from build123d import *

# Parameters (mm, degrees)
SKETCH1_R                      = 5.556
EXTRUDE1_DEPTH                 = 100.645
THREADCHAMFER_SIZE             = 1.2
SKETCH3_OUTSIDE_W              = 33.484
SKETCH3_OUTSIDE_H              = 33.484
SKETCH3_OUTSIDE_R              = 5.1
CUT_EXTRUDE1_DEPTH             = 2
CHAMFER2_SIZE                  = 0.3
SKETCH4_R                      = 15.8
PISTON_DEPTH                   = 5
CUT_EXTRUDE2_REACH             = 105.096
CUT_EXTRUDE2_DIRECTION_2_REACH = 105.096


with BuildPart() as part:
    # Sketch1 → Extrude1 (new body)
    with BuildSketch(Plane.XY):
        with Locations(Location((0, 0, 0), (0, 0, 90))):
            Circle(SKETCH1_R)
    extrude(amount=EXTRUDE1_DEPTH)

    # ThreadChamfer
    threadchamfer_edges = [part.edges().sort_by_distance(p)[0] for p in [
        (0, -5.556, 100.645),
    ]]
    chamfer(threadchamfer_edges, length=THREADCHAMFER_SIZE)

    # Sketch3 outside → Cut-Extrude1 (cut)
    with BuildSketch(Plane.XY.offset(81.645)):
        Rectangle(SKETCH3_OUTSIDE_W, SKETCH3_OUTSIDE_H)
        Circle(SKETCH3_OUTSIDE_R, mode=Mode.SUBTRACT)
    extrude(amount=-CUT_EXTRUDE1_DEPTH, mode=Mode.SUBTRACT)

    # Chamfer2
    chamfer2_edges = [part.edges().sort_by_distance(p)[0] for p in [
        (0, -5.556, 79.645),
    ]]
    chamfer(chamfer2_edges, length=CHAMFER2_SIZE)

    # Sketch4 → Piston (add)
    with BuildSketch(Plane.XY):
        Circle(SKETCH4_R)
    extrude(amount=PISTON_DEPTH)

    # Sketch5 → Cut-Extrude2 (cut, up to next)
    with BuildSketch(Plane(origin=(0, 0, 0), x_dir=(1, 0, 0), z_dir=(0, 1, 0)), mode=Mode.PRIVATE) as cut_extrude2_sk1:
        Polygon((5.556, -75.565), (4.826, -76.295), (4.826, -82.645), (5.556, -83.375), align=None)
    cut_extrude2_tool1 = extrude(cut_extrude2_sk1.sketch, amount=-CUT_EXTRUDE2_REACH, mode=Mode.PRIVATE) & part.part
    # Sketch5 → Cut-Extrude2 (cut, up to next)
    with BuildSketch(Plane(origin=(0, 0, 0), x_dir=(1, 0, 0), z_dir=(0, 1, 0)), mode=Mode.PRIVATE) as cut_extrude2_sk2:
        Polygon((-5.556, -83.375), (-4.826, -82.645), (-4.826, -76.295), (-5.556, -75.565), align=None)
    cut_extrude2_tool2 = extrude(cut_extrude2_sk2.sketch, amount=-CUT_EXTRUDE2_REACH, mode=Mode.PRIVATE) & part.part
    add(cut_extrude2_tool1.solids().sort_by_distance((5.203545, 0, 79.47))[0], mode=Mode.SUBTRACT)
    add(cut_extrude2_tool2.solids().sort_by_distance((-5.203545, 0, 79.47))[0], mode=Mode.SUBTRACT)

    # Sketch5 → Cut-Extrude2 direction 2 (cut, up to next)
    with BuildSketch(Plane(origin=(0, 0, 0), x_dir=(1, 0, 0), z_dir=(0, 1, 0)), mode=Mode.PRIVATE) as cut_extrude2_direction_2_sk1:
        Polygon((5.556, -75.565), (4.826, -76.295), (4.826, -82.645), (5.556, -83.375), align=None)
    cut_extrude2_direction_2_tool1 = extrude(cut_extrude2_direction_2_sk1.sketch, amount=CUT_EXTRUDE2_DIRECTION_2_REACH, mode=Mode.PRIVATE) & part.part
    # Sketch5 → Cut-Extrude2 direction 2 (cut, up to next)
    with BuildSketch(Plane(origin=(0, 0, 0), x_dir=(1, 0, 0), z_dir=(0, 1, 0)), mode=Mode.PRIVATE) as cut_extrude2_direction_2_sk2:
        Polygon((-5.556, -83.375), (-4.826, -82.645), (-4.826, -76.295), (-5.556, -75.565), align=None)
    cut_extrude2_direction_2_tool2 = extrude(cut_extrude2_direction_2_sk2.sketch, amount=CUT_EXTRUDE2_DIRECTION_2_REACH, mode=Mode.PRIVATE) & part.part
    add(cut_extrude2_direction_2_tool1.solids().sort_by_distance((5.203545, 0, 79.47))[0], mode=Mode.SUBTRACT)
    add(cut_extrude2_direction_2_tool2.solids().sort_by_distance((-5.203545, 0, 79.47))[0], mode=Mode.SUBTRACT)


solid = part.part
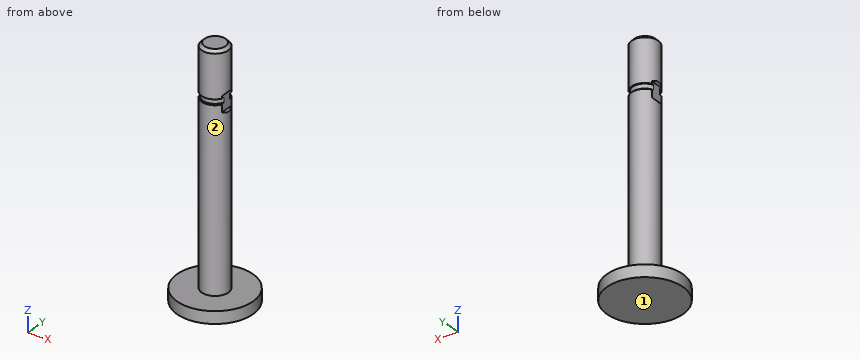
Part model, mm, in its own coordinate system. Face numbers are marked on the shaded views. A direction names the side the tool comes from. Give positions to 0.01 mm unless a question says otherwise; leave off trailing zeros. Write each loop counter-clockwise with the first axis right and the second up, starting at its lowest first coordinate (ties: lowest second). Pieces come first, ordered by that corner, then holes.
1) Pin check, flat tips, straight feed: pin 1 (4.5 mm diameter, centred on y = -1, z = 79, fed in from +X); pin 2 (12 mm diameter, centred on y = 7.5, z = 46.5, fed in from -X); pin 3 (3 mm diameter, centred on y = 1, z = 79.5, fed in from -X). Stop position of each tip, or through.
Resolved:
pin 1: stops at x = 4.83
pin 2: stops at x = -5.35
pin 3: stops at x = -4.83
2) Cut at D-D on y = -7. Write the cut outline in (x, z), then the cut area to 3 significant figures.
Resolved:
outline: (-14.16, 0) - (14.16, 0) - (14.16, 5) - (-14.16, 5) - close
area: 142 mm2
3) Probe L1, parallel to X at y = 0, z = 78; L2, parallel to Z at x = 7, y = 3.5; L3, parallel to Y at x = 0.5, z = 57.5. List the from-to ranges inside material, lowest first.
Resolved:
L1: x = -4.83 to 4.83
L2: z = 0 to 5
L3: y = -5.53 to 5.53
4) Cut at C-C on z = 6.5. Write the cut outline in (x, y), then the cut area to 3 significant figures.
Resolved:
outline: circle Ø11.11 at (0, 0)
area: 97.0 mm2
5) Cut at A-A on y = 0. Write the cut outline in (x, z) (3 decimals), then the cut area to 3 significant figures.
Resolved:
outline: (-15.8, 0) - (15.8, 0) - (15.8, 5) - (5.556, 5) - (5.556, 75.565) - (4.826, 76.295) - (4.826, 82.645) - (5.556, 83.375) - (5.556, 99.445) - (4.356, 100.645) - (-4.356, 100.645) - (-5.556, 99.445) - (-5.556, 83.375) - (-4.826, 82.645) - (-4.826, 76.295) - (-5.556, 75.565) - (-5.556, 5) - (-15.8, 5) - close
area: 1,210 mm2
6) Which spindle directions (+Z, -Z, +X, -X, +Y, -Y) get a long thin tool onto all of the face, cutting with end or side? Do the marked faces 1 and 2. Say none if no direction does.
Resolved:
face 1: -Z, +X, -X, +Y, -Y
face 2: +Z
7) Cut at B-B on x = 0. Write the cut outline in (y, z) (3 decimals), then the cut area to 3 significant figures.
Resolved:
outline: (-15.8, 0) - (15.8, 0) - (15.8, 5) - (5.556, 5) - (5.556, 79.345) - (5.256, 79.645) - (5.1, 79.645) - (5.1, 81.645) - (5.556, 81.645) - (5.556, 99.445) - (4.356, 100.645) - (-4.356, 100.645) - (-5.556, 99.445) - (-5.556, 81.645) - (-5.1, 81.645) - (-5.1, 79.645) - (-5.256, 79.645) - (-5.556, 79.345) - (-5.556, 5) - (-15.8, 5) - close
area: 1,220 mm2
